Here's the drawing with two shaded views (mm, measured from the low corner). I have some questions. A direction names the side the tool comes from. Give positions to 0.01 mm unless a question says otherwise; leave off trailing zeros. Loops run counter-clockwise (first coordinate to the right, second up) from the corner with the lowest first, then second, coordinate; pieces in that order, holes last. Notation, with made-up numbers: (42.25, -9) -> (60.25, -9) arc R7 ccw to (60.25, 3) -> close; hole circle Ø10 at (40, 66). An arc over 180 degrees is marked (long way). Put each result on its own line as item: value.
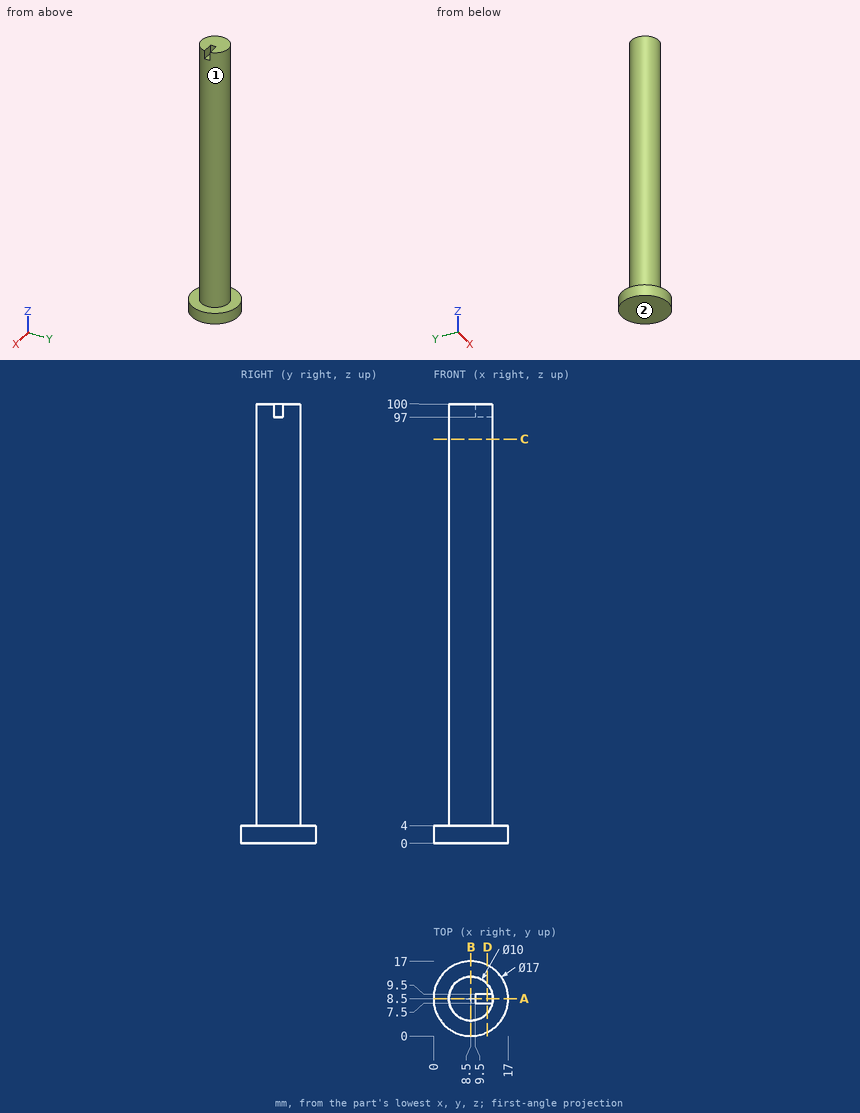
1. If we section it at C-C (z = 92): List the corners of the cut face in (x, y) for me, then the cut area to 3 significant figures.
Recorded:
outline: circle Ø10 at (8.5, 8.5)
area: 78.5 mm^2
2. If we section it at D-D (x = 12.25): List the corners of the cut face in (y, z) for me.
Recorded:
outline: (0.87, 0) -> (16.13, 0) -> (16.13, 4) -> (11.81, 4) -> (11.81, 100) -> (9.5, 100) -> (9.5, 97) -> (7.5, 97) -> (7.5, 100) -> (5.19, 100) -> (5.19, 4) -> (0.87, 4) -> close
3. I need wall thicknesses on line 1 (Z direction, x = 15.25, y = 7.25); line 2 (X direction, y = 8.75, z = 37); line 3 (Y direction, x = 8, z = 57.5). Which ranges of each line are inside material? Lowest first, please.
Recorded:
line 1: z = 0 to 4
line 2: x = 3.51 to 13.49
line 3: y = 3.53 to 13.47
4. I'm going to push flat-ended pins straight in: pin 1 (1.6 mm diameter, centred on y = 8, z = 98, fed in from +X); pin 2 (1.5 mm diameter, centred on x = 2.5, y = 6.5, fed in from -Z); pin 3 (8 mm diameter, centred on y = 2, z = 29.5, fed in from +X); pin 4 (6 mm diameter, centred on y = 3, z = 56, fed in from -X). Where does each tip first touch, or does it pass through?
Recorded:
pin 1: stops at x = 13.4
pin 2: stops at z = 0
pin 3: stops at x = 12.83
pin 4: stops at x = 4.17
5. If we section it at B-B (x = 8.5): List the corners of the cut face in (y, z) for me, then the cut area to 3 significant figures.
Recorded:
outline: (0, 0) -> (17, 0) -> (17, 4) -> (13.5, 4) -> (13.5, 100) -> (3.5, 100) -> (3.5, 4) -> (0, 4) -> close
area: 1,030 mm^2
6. If we section it at A-A (y = 8.5): List the corners of the cut face in (x, z) for me.
Recorded:
outline: (0, 0) -> (17, 0) -> (17, 4) -> (13.5, 4) -> (13.5, 97) -> (9.5, 97) -> (9.5, 100) -> (3.5, 100) -> (3.5, 4) -> (0, 4) -> close
7. For the marked faces 1 and 2, which set-ups out of +Z, -Z, +X, -X, +Y, -Y let a thin tool reach every point of the face, with its end or its side?
Recorded:
face 1: +Z
face 2: -Z, +X, -X, +Y, -Y
